Can you work these out from the model? Positions are in its coordinate system, mm. Face numbers are marked on the shaded views. A direction names the side the tool comes from. Coordinates: 2 decimals unless noted, no trailing zeros. Write each loop counter-clockwise with the first axis right and the second up, starting at its lowest first coordinate (ties: lowest second). Pieces come first, ordered by that corner, then holes. Notation, with made-up numbers: M 4.5,48.25 L 42.5,48.25 A24 cw 42.5,82.25 Z; hole C -39.75,43.5 d6. An arc over 180 degrees is marked long. Answer as a JSON object with one key per item and string values. Group by question number.
from build123d import *

# Parameters (mm, degrees)
BOSS_EXTRUDE1_DEPTH = 50
SKETCH2_R           = 2.25
CUT_EXTRUDE1_DEPTH  = 24
CUT_EXTRUDE2_REACH  = 4
SKETCH3_R           = 2.25


with BuildPart() as part:
    # Sketch1 → Boss-Extrude1 (new body)
    with BuildSketch(Plane.XY):
        with BuildLine():
            Line((0, 12), (10, 12))
            Line((10, 12), (10, 27))
            Line((10, 27), (12, 27))
            Line((12, 27), (12, 10))
            Line((12, 10), (0, 10))
            ThreePointArc((0, 10), (-10, 0), (0, -10))
            Line((0, -10), (12, -10))
            Line((12, -10), (12, -27))
            Line((12, -27), (10, -27))
            Line((10, -27), (10, -12))
            Line((10, -12), (0, -12))
            ThreePointArc((0, -12), (-12, 0), (0, 12))
        make_face()
    extrude(amount=BOSS_EXTRUDE1_DEPTH)

    # Sketch2 → Cut-Extrude1 (cut)
    with BuildSketch(Plane(origin=(0, 12, 0), x_dir=(1, 0, 0), z_dir=(0, 1, 0))):
        with Locations((0, -25)):
            Circle(SKETCH2_R)
    extrude(amount=-CUT_EXTRUDE1_DEPTH, mode=Mode.SUBTRACT)

    # Sketch3 → Cut-Extrude2 (cut, up to next)
    with BuildSketch(Plane.ZY.offset(-10), mode=Mode.PRIVATE) as cut_extrude2_sk1:
        with Locations((10, 19.5)):
            Circle(SKETCH3_R)
    cut_extrude2_tool1 = extrude(cut_extrude2_sk1.sketch, amount=-CUT_EXTRUDE2_REACH, mode=Mode.PRIVATE) & part.part
    add(cut_extrude2_tool1.solids().sort_by_distance((10, 19.5, 10))[0], mode=Mode.SUBTRACT)
    # Sketch3 → Cut-Extrude2 (cut, up to next)
    with BuildSketch(Plane.ZY.offset(-10), mode=Mode.PRIVATE) as cut_extrude2_sk2:
        with Locations((40, 19.5)):
            Circle(SKETCH3_R)
    cut_extrude2_tool2 = extrude(cut_extrude2_sk2.sketch, amount=-CUT_EXTRUDE2_REACH, mode=Mode.PRIVATE) & part.part
    add(cut_extrude2_tool2.solids().sort_by_distance((10, 19.5, 40))[0], mode=Mode.SUBTRACT)
    # Sketch3 → Cut-Extrude2 (cut, up to next)
    with BuildSketch(Plane.ZY.offset(-10), mode=Mode.PRIVATE) as cut_extrude2_sk3:
        with Locations((40, -19.5)):
            Circle(SKETCH3_R)
    cut_extrude2_tool3 = extrude(cut_extrude2_sk3.sketch, amount=-CUT_EXTRUDE2_REACH, mode=Mode.PRIVATE) & part.part
    add(cut_extrude2_tool3.solids().sort_by_distance((10, -19.5, 40))[0], mode=Mode.SUBTRACT)
    # Sketch3 → Cut-Extrude2 (cut, up to next)
    with BuildSketch(Plane.ZY.offset(-10), mode=Mode.PRIVATE) as cut_extrude2_sk4:
        with Locations((10, -19.5)):
            Circle(SKETCH3_R)
    cut_extrude2_tool4 = extrude(cut_extrude2_sk4.sketch, amount=-CUT_EXTRUDE2_REACH, mode=Mode.PRIVATE) & part.part
    add(cut_extrude2_tool4.solids().sort_by_distance((10, -19.5, 10))[0], mode=Mode.SUBTRACT)


solid = part.part
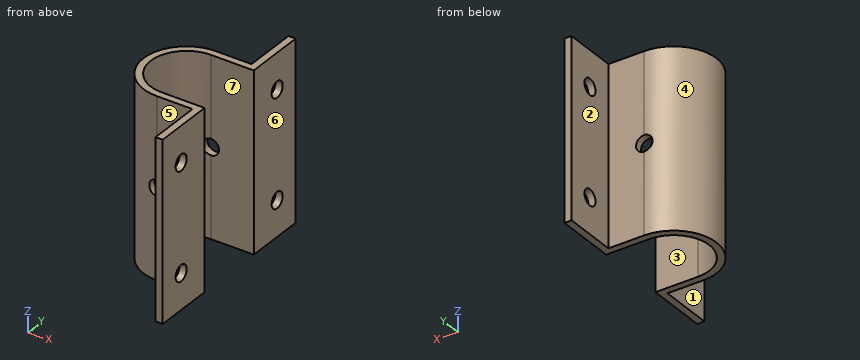
Q1. Please list where these lines run through material, in increasing order: L1, parallel to Y at x = 10.6, z = 40; L2, parallel to Z at x = 0, y = 11.15; L3, parallel to Y at x = 8.5, z = 19.
Q2. If we section it at D-D on z = 45: List the corners of the cut face in (x, y) for me, and give its area (3 significant figures).
Q3. We'd pull the mould along Y, two halves only. Please class the marked faces 5, 6 and 7: pulls with the +Y half, pulls with the -Y half, needs draft (parallel to the pull), parting line crosses it, or undercut.
Q4. On a 3-axis mill with a long thin cutter (end or side, diameter ignored), from which of +Z, -Z, +X, -X, +Y, -Y can I reach the whole of each face in a straight line? I mean the marked faces 1, 2, 3 and 4. Say none if no direction works.
Q5. Will these pins go through, and if not, where does the flat tip stop? pin 1 (3 mm diameter, centred on y = -1.5, z = 21, fed in from +X); pin 2 (6 mm diameter, centred on x = 0, z = 25, fed in from -Y); pin 3 (9.5 mm diameter, centred on x = 3.5, z = 22, fed in from +Y).
Q6. If we section it at A-A on z = 10: List the corners of the cut face in (x, y) for me.
Q7. If we section it at C-C on y = -19.5: List the corners of the cut face in (x, z) for me.
Q8. If we section it at B-B on x = 9: List the corners of the cut face in (y, z) for me, and give its area (3 significant figures).
Reply:
{
 "1": {"L1": "-27 to -21.75, -17.25 to -10, 10 to 17.25, 21.75 to 27", "L2": "0 to 22.75, 27.25 to 50", "L3": "-12 to -10, 10 to 12"},
 "2": {"outline": "M 0,-12 L 10,-12 L 10,-27 L 12,-27 L 12,-10 L 0,-10 A10 cw 0,10 L 12,10 L 12,27 L 10,27 L 10,12 L 0,12 A12 ccw Z", "area": "177 mm^2"},
 "3": {"face 5": "pulls with the -Y half", "face 6": "needs draft", "face 7": "undercut"},
 "4": {"face 1": "+Z, -Z, -X, -Y", "face 2": "+Z, -Z, -X, +Y", "face 3": "+Z, -Z, +X", "face 4": "+Z, -Z, -X"},
 "5": {"pin 1": "x = -9.54", "pin 2": "y = -12", "pin 3": "y = 12"},
 "6": {"outline": "M 0,-12 L 10,-12 L 10,-17.25 L 12,-17.25 L 12,-10 L 0,-10 A10 cw 0,10 L 12,10 L 12,17.25 L 10,17.25 L 10,12 L 0,12 A12 ccw Z; M 10,-27 L 12,-27 L 12,-21.75 L 10,-21.75 Z; M 10,21.75 L 12,21.75 L 12,27 L 10,27 Z"},
 "7": {"outline": "M 10,0 L 12,0 L 12,7.75 L 10,7.75 Z; M 10,12.25 L 12,12.25 L 12,37.75 L 10,37.75 Z; M 10,42.25 L 12,42.25 L 12,50 L 10,50 Z"},
 "8": {"outline": "M -12,0 L -10,0 L -10,50 L -12,50 Z; M 10,0 L 12,0 L 12,50 L 10,50 Z", "area": "200 mm^2"}
}
